Read the model definition and answer for the solid it produces. Units are mm, in the model's axes. A direction names the side the tool comes from. Give positions to 0.01 mm unless a question says otherwise; leave off trailing zeros. Order: outer loops, then holes, each group sorted by start corner. A loop starts at its lowest first (then second) coordinate and runs counter-clockwise, first axis right, second up. Notation, with made-up numbers: (39, 62.25) -> (79, 62.25) arc R18 ccw to (79, 93.25) -> close; hole circle Ø2 at (7, 1.5). An arc over 180 degrees is marked (long way). Use one line per item in the form item = value.
```python
from build123d import *

# Parameters (mm, degrees)
F1_DEPTH = 23.3
F2_W     = 44.94
F2_H     = 0.25
F3_DEPTH = 12.281
F4_W     = 5.45
F4_H     = 1.23
F5_DEPTH = 5.4


with BuildPart() as f1:
    # F0 (on Right) → F1 (new body, symmetric)
    with BuildSketch(Plane.YZ):
        Polygon((-0.24, 14.18), (-6.14, 14.18), (-6.14, 0), (6.14, 0), (6.14, 13.3), (0.73, 13.3), align=None)
    extrude(amount=F1_DEPTH, both=True)

    # F2 (on face) → F3 (cut, through all)
    with BuildSketch(Plane.XZ.offset(6.14)):
        with Locations((0, 0.125)):
            Rectangle(F2_W, F2_H)
    extrude(amount=-F3_DEPTH, mode=Mode.SUBTRACT)

    # F4 (on face) → F5 (cut)
    with BuildSketch(Plane.XZ.offset(6.14)):
        Polygon((-12.15, 5.822), (-20.9, 5.822), (-20.9, 1.122), (-12.15, 1.122), (-12.15, 2.372), (-11.15, 2.372), (-11.15, 4.572), (-12.15, 4.572), align=None)
        with Locations((-16.525, 3.957)):
            Rectangle(F4_W, F4_H, mode=Mode.SUBTRACT)
        Polygon((-9.975, 5.822), (-9.975, 1.122), (3.875, 1.122), (3.875, 2.372), (4.875, 2.372), (4.875, 4.572), (3.875, 4.572), (3.875, 5.822), align=None)
        Polygon((-8.215, 2.372), (-8.215, 4.572), (2.195, 4.572), (2.195, 3.342), (-7.065, 3.342), (-7.065, 2.372), align=None, mode=Mode.SUBTRACT)
        Polygon((6.05, 5.822), (6.05, 1.122), (19.9, 1.122), (19.9, 2.372), (20.9, 2.372), (20.9, 4.572), (19.9, 4.572), (19.9, 5.822), align=None)
        Polygon((7.81, 2.372), (7.81, 4.572), (18.22, 4.572), (18.22, 3.342), (8.96, 3.342), (8.96, 2.372), align=None, mode=Mode.SUBTRACT)
        Polygon((6.05, 8.48), (19.9, 8.48), (19.9, 9.73), (20.9, 9.73), (20.9, 11.93), (19.9, 11.93), (19.9, 13.18), (6.05, 13.18), align=None)
        Polygon((7.81, 11.822), (18.22, 11.822), (18.22, 10.592), (8.96, 10.592), (8.96, 9.622), (7.81, 9.622), align=None, mode=Mode.SUBTRACT)
        Polygon((3.875, 11.93), (3.875, 13.18), (-9.975, 13.18), (-9.975, 8.48), (3.875, 8.48), (3.875, 9.73), (4.875, 9.73), (4.875, 11.93), align=None)
        Polygon((-8.215, 11.822), (2.195, 11.822), (2.195, 10.592), (-7.065, 10.592), (-7.065, 9.622), (-8.215, 9.622), align=None, mode=Mode.SUBTRACT)
        Polygon((-12.15, 11.93), (-12.15, 13.18), (-20.9, 13.18), (-20.9, 8.48), (-12.15, 8.48), (-12.15, 9.73), (-11.15, 9.73), (-11.15, 11.93), align=None)
        with Locations((-16.525, 11.207)):
            Rectangle(F4_W, F4_H, mode=Mode.SUBTRACT)
    extrude(amount=-F5_DEPTH, mode=Mode.SUBTRACT)


solid = f1.part
```
Item 1: The part is cut by section A-A on x = -13. Give the vertices of the cut face in (y, z), and give its area (3 significant figures).
Checks:
outline = (-6.14, 0.25) -> (6.14, 0.25) -> (6.14, 13.3) -> (0.73, 13.3) -> (-0.24, 14.18) -> (-6.14, 14.18) -> (-6.14, 13.18) -> (-0.74, 13.18) -> (-0.74, 8.48) -> (-6.14, 8.48) -> (-6.14, 5.82) -> (-0.74, 5.82) -> (-0.74, 1.12) -> (-6.14, 1.12) -> close
area = 115 mm²
Item 2: The part is cut by section C-C on z = 11. Give the vertices of the cut face in (x, y) (3 decimals), and give its area (3 significant figures).
Checks:
outline = (-23.3, -6.14) -> (-20.9, -6.14) -> (-20.9, -0.74) -> (-19.25, -0.74) -> (-19.25, -6.14) -> (-13.8, -6.14) -> (-13.8, -0.74) -> (-11.15, -0.74) -> (-11.15, -6.14) -> (-9.975, -6.14) -> (-9.975, -0.74) -> (-8.215, -0.74) -> (-8.215, -6.14) -> (2.195, -6.14) -> (2.195, -0.74) -> (4.875, -0.74) -> (4.875, -6.14) -> (6.05, -6.14) -> (6.05, -0.74) -> (7.81, -0.74) -> (7.81, -6.14) -> (18.22, -6.14) -> (18.22, -0.74) -> (20.9, -0.74) -> (20.9, -6.14) -> (23.3, -6.14) -> (23.3, 6.14) -> (-23.3, 6.14) -> close
area = 501 mm²
Item 3: Given pin 1 Ø1 at (x, y) = (12.5, -4) entering from -Z, flat-ended and moving along its own axis, determine where the tip first touches the part or whether it passes through.
Checks:
pin_1 = 0.25
Item 4: Determine the mould class of faces 1 (the flat face through (-3, -6.14, 11)), 2 (the flat face through (-13.8, -3, 4)), 3 (the flat face through (-17, -3, 4.572)) for opening direction Z: +Z half, -Z half, draft (parallel to the pull), parting line (faces both ways), or undercut.
Checks:
face_1 = draft
face_2 = undercut
face_3 = undercut
Item 5: The part is cut by section D-D on y = 2. Give the vertices of the cut face in (x, z), and give its area (3 significant figures).
Checks:
outline = (-23.3, 0) -> (-22.47, 0) -> (-22.47, 0.25) -> (22.47, 0.25) -> (22.47, 0) -> (23.3, 0) -> (23.3, 13.3) -> (-23.3, 13.3) -> close
area = 609 mm²
Item 6: Which of the six approach directions +Z, -Z, +X, -X, +Y, -Y give full straight-line access (tool end or side, diameter ignored) to faces 4 (the flat face through (-17, -3, 8.48)), 5 (the flat face through (0, -6.14, 7))?
Checks:
face_4 = -Y
face_5 = +Z, -Z, +X, -X, -Y
Item 7: The part is cut by section B-B on y = -2. State how many separate pieces and enclosed holes the cut face has, and give its area (3 significant figures).
Checks:
separate_pieces = 7
enclosed_holes = 6
area = 363 mm²
Item 8: Straight lines are drawn through the part: L1, parallel to Z at x = -19.5, y = -1.75; L2, parallel to X at y = -5, z = 9.5 (3 decimals); L3, parallel to Z at x = -5.5, y = -2.75. For each, find the intervals that lie inside material, in ascending order. Write a range as from..to.
Checks:
L1 = 0.25..1.12, 5.82..8.48, 13.18..14.18
L2 = -23.3..-20.9, -12.15..-9.975, 3.875..6.05, 19.9..23.3
L3 = 0.25..1.12, 3.34..4.57, 5.82..8.48, 10.59..11.82, 13.18..14.18
